```python
from build123d import *

# Parameters (mm, degrees)
BASE_FLANGIA1_DEPTH            = 2
BORDO_FLANGIA1_STRIP_W         = 11
BORDO_FLANGIA1_STRIP_H         = 2
BORDO_FLANGIA1_STRIP_CUT_DEPTH = 58
BORDO_FLANGIA1_DEPTH           = 58
BORDO_FLANGIA2_STRIP_W         = 11
BORDO_FLANGIA2_STRIP_H         = 2
BORDO_FLANGIA2_STRIP_CUT_DEPTH = 58
BORDO_FLANGIA2_DEPTH           = 58
SCHIZZO11_R                    = 3
TAGLIO_ESTRUSIONE1_DEPTH       = 50
RACCORDO2_R                    = 1
SCHIZZO16_R                    = 4.25
TAGLIO_ESTRUSIONE2_DEPTH       = 10


# Sheet-metal steps are written as plain solids
with BuildPart() as part:
    # Schizzo1 → Base-Flangia1 (new body)
    with BuildSketch(Plane(origin=(0, 0, 0), x_dir=(1, 0, 0), z_dir=(0, 1, 0))):
        Polygon((0, 0), (-6, 0), (-16, 0), (-22, 0), (-22, 58), (0, 58), align=None)
    extrude(amount=-BASE_FLANGIA1_DEPTH)

    # Bordo-Flangia1 strip (across the edge) → Bordo-Flangia1 strip cut (cut)
    with BuildSketch(Plane(origin=(-22, 0, -58), x_dir=(1, 0, 0), z_dir=(0, 0, 1))):
        with Locations((-4, -1)):
            Rectangle(BORDO_FLANGIA1_STRIP_W, BORDO_FLANGIA1_STRIP_H)
    extrude(amount=BORDO_FLANGIA1_STRIP_CUT_DEPTH, mode=Mode.SUBTRACT)

    # Bordo-Flangia1 section (across the edge) → Bordo-Flangia1 (add)
    with BuildSketch(Plane(origin=(-22, 0, -58), x_dir=(1, 0, 0), z_dir=(0, 0, 1))):
        with BuildLine():
            Line((-2, 1.5), (-2, 42))
            Line((-2, 42), (0, 42))
            Line((0, 42), (0, 1.5))
            ThreePointArc((0, 1.5), (0.439339828, 0.439339828), (1.5, 0))
            Line((1.5, 0), (1.5, -2))
            ThreePointArc((1.5, -2), (-0.974873734, -0.974873734), (-2, 1.5))
        make_face()
    extrude(amount=BORDO_FLANGIA1_DEPTH)

    # Bordo-Flangia2 strip (across the edge) → Bordo-Flangia2 strip cut (cut)
    with BuildSketch(Plane(origin=(0, 0, 0), x_dir=(-1, 0, 0), z_dir=(0, 0, -1))):
        with Locations((-4, -1)):
            Rectangle(BORDO_FLANGIA2_STRIP_W, BORDO_FLANGIA2_STRIP_H)
    extrude(amount=BORDO_FLANGIA2_STRIP_CUT_DEPTH, mode=Mode.SUBTRACT)

    # Bordo-Flangia2 section (across the edge) → Bordo-Flangia2 (add)
    with BuildSketch(Plane(origin=(0, 0, 0), x_dir=(-1, 0, 0), z_dir=(0, 0, -1))):
        with BuildLine():
            Line((-2, 1.5), (-2, 42))
            Line((-2, 42), (0, 42))
            Line((0, 42), (0, 1.5))
            ThreePointArc((0, 1.5), (0.439339828, 0.439339828), (1.5, 0))
            Line((1.5, 0), (1.5, -2))
            ThreePointArc((1.5, -2), (-0.974873734, -0.974873734), (-2, 1.5))
        make_face()
    extrude(amount=BORDO_FLANGIA2_DEPTH)

    # Schizzo11 → Taglio-Estrusione1 (cut)
    with BuildSketch(Plane.ZY.offset(24)):
        with BuildLine():
            Line((-58, 42), (-58, 36.5))
            ThreePointArc((-58, 36.5), (-56.389087297, 40.389087297), (-52.5, 42))
            Line((-52.5, 42), (-58, 42))
        make_face()
        with BuildLine():
            Line((-50.048262739, 41.42331031), (0, 16.5))
            Line((0, 16.5), (0, 42))
            Line((0, 42), (-52.5, 42))
            ThreePointArc((-52.5, 42), (-51.240676114, 41.853886752), (-50.048262739, 41.42331031))
        make_face()
        with Locations(Location((-52.5, 36.5, 0), (0, 0, 270))):
            Circle(SCHIZZO11_R)
    extrude(amount=-TAGLIO_ESTRUSIONE1_DEPTH, mode=Mode.SUBTRACT)

    # Raccordo2
    raccordo2_edges = [part.edges().sort_by_distance(p)[0] for p in [
        (1, 16.5, 0),
        (-23, 16.5, 0),
    ]]
    fillet(raccordo2_edges, radius=RACCORDO2_R)

    # Schizzo16 → Taglio-Estrusione2 (cut)
    with BuildSketch(Plane.XZ.offset(2)):
        with Locations(Location((-11, -45.75, 0), (0, 0, 270))):
            Circle(SCHIZZO16_R)
        with BuildLine():
            Line((-15.25, -9.75), (-16, 0))
            Line((-16, 0), (-6, 0))
            Line((-6, 0), (-6.75, -9.75))
            ThreePointArc((-6.75, -9.75), (-11, -14), (-15.25, -9.75))
        make_face()
    extrude(amount=-TAGLIO_ESTRUSIONE2_DEPTH, mode=Mode.SUBTRACT)


solid = part.part
```
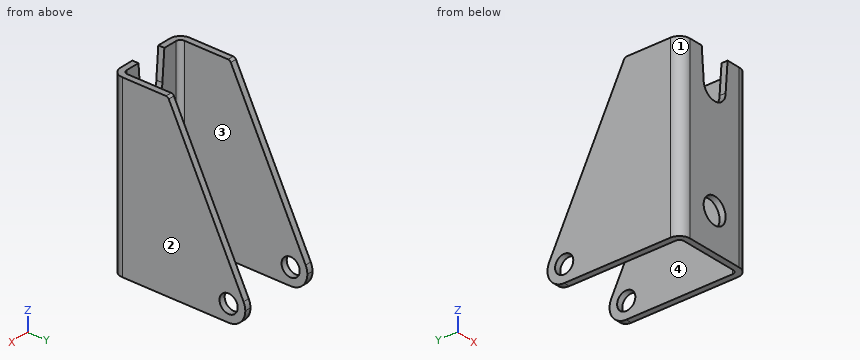
For this review, take the finished solid that the model builds, in its own axes (mm). Face numbers are marked on the shaded views. Give positions to 0.01 mm unless a question says otherwise; leave off trailing zeros. Write each loop counter-clockwise with the first axis right and the second up, starting at its lowest first coordinate (ties: lowest second). Pieces come first, ordered by that corner, then holes.
Item 1: Take a section at B-B (y = 7.5). Give the boundary of the cut face in (x, z).
Item 2: Insertion check: P1, Ø12, axis at x = -15.5, z = -42.5, coming from the +Y side; P2, Ø3, axis at x = -14, z = -26, coming from the +Y side; P3, Ø4, axis at x = -21, z = -28.5, coming from the +Y side. Each pin has a flat end and moves straight along its axis. Give the tip position at first contact, or say it passes through.
Item 3: Wall thickness on probe 1 along X at (y, z) = (13, -29.5); probe 2 along Y at (x, z) = (-9.25, -34); probe 3 along Z at (x, y) = (1, 36.5): over which ranges is each line inside the solid? List them lowest first.
Item 4: Take a section at D-D (z = -45.75). Give the boundary of the cut face in (x, y).
Item 5: Take a section at A-A (x = -11). Give the boundary of the cut face in (y, z).
Item 6: Take a section at C-C (y = 34.5). Give the boundary of the cut face in (x, z).
Item 7: The part is to be moulded in two halves that separate along X. For the marked faces 1, 2, 3 and 4, say which applies: +X half, -X half, draft (parallel to the pull), parting line (faces both ways), or undercut.
Established:
1. outline: (-24, -58) - (-22, -58) - (-22, 0) - (-24, 0) - close; (0, -58) - (2, -58) - (2, 0) - (0, 0) - close
2. P1: stops at y = 0.38
2. P2: stops at y = 0
2. P3: stops at y = 31.56
3. probe 1: x = -24 to -22, 0 to 2
3. probe 2: y = -2 to 0
3. probe 3: z = -58 to -55.5, -49.5 to -40.16
4. outline: (-24, 1.5) arc R3.5 ccw to (-20.5, -2) - (-15.25, -2) - (-15.25, 0) - (-20.5, 0) arc R1.5 cw to (-22, 1.5) - (-22, 39.28) - (-24, 39.28) - close; (-6.75, -2) - (-1.5, -2) arc R3.5 ccw to (2, 1.5) - (2, 39.28) - (0, 39.28) - (0, 1.5) arc R1.5 cw to (-1.5, 0) - (-6.75, 0) - close
5. outline: (-2, -58) - (0, -58) - (0, -50) - (-2, -50) - close; (-2, -41.5) - (0, -41.5) - (0, -14) - (-2, -14) - close
6. outline: (-24, -58) - (-22, -58) - (-22, -54.74) - (-24, -54.74) - close; (-24, -50.26) - (-22, -50.26) - (-22, -36.15) - (-24, -36.15) - close; (0, -58) - (2, -58) - (2, -54.74) - (0, -54.74) - close; (0, -50.26) - (2, -50.26) - (2, -36.15) - (0, -36.15) - close
7. face 1: -X half
7. face 2: +X half
7. face 3: undercut
7. face 4: undercut
